Read the model definition and answer for the solid it produces. Units are mm, in the model's axes. Face numbers are marked on the shaded views. A direction names the side the tool comes from. Give positions to 0.01 mm unless a question says otherwise; leave off trailing zeros. Order: outer loops, then holes, each group sorted by start corner. A loop starts at its lowest first (then second) coordinate and runs counter-clockwise, first axis right, second up. Notation, with made-up numbers: (73, 54) - (132, 54) arc R22 ccw to (132, 73) - close; hole circle Ø1 at (20, -11). An arc over 180 degrees is marked (long way). Write each question's results on one line, items separated by ' | '.
Autodesk Inventor part; units mm, degrees
ref_plane "YZ Plane" through (0, 0, 0) normal (1, 0, 0) x (0, 1, 0)
ref_plane "XZ Plane" through (0, 0, 0) normal (0, 1, 0) x (-1, 0, 0)
ref_plane "XY Plane" through (0, 0, 0) normal (0, 0, 1) x (1, 0, 0)
sketch "Sketch1" plane through (0, 0, 0) normal (0, 1, 0) x (-1, 0, 0)
  circle A0 centre (0, 0) radius 5.5
  dimension "d0" = 11
extrude "Extrusion1" add sketch "Sketch1" along normal blind 33
sketch "Sketch6" plane through (0, 0, 0) normal (0, -1, 0) x (1, 0, 0)
  circle A0 centre (0, 0) radius 5.5
  line L0 (3.45, 0) -> (3.45, -4.2834)
  line L1 (0.45, 0) -> (0.45, -5.4816)
  line L2 (3.45, -5.4816) -> (3.45, -4.2834)
  line L3 (3.45, -5.4816) -> (0.45, -5.4816)
  line L4 (0.45, 0) -> (0.45, 5.4816)
  line L5 (3.45, 5.3243) -> (3.45, 0)
  line L6 (3.45, 5.3243) -> (0.45, 5.4816)
  line L7 (0, -5.5) -> (0, 5.5)
  line L8 (-3.45, 0) -> (-3.45, -4.2834)
  line L9 (-0.45, 0) -> (-0.45, -5.4816)
  line L10 (-3.45, -5.4816) -> (-3.45, -4.2834)
  line L11 (-3.45, -5.4816) -> (-0.45, -5.4816)
  line L12 (-0.45, 0) -> (-0.45, 5.4816)
  line L13 (-3.45, 5.3243) -> (-3.45, 0)
  line L14 (-3.45, 5.3243) -> (-0.45, 5.4816)
  point P0 (-3.45, 4.2834)
  point P1 (3.45, 4.2834)
  dimension "d20" = 3
  dimension "d21" = 3
  dimension "d22" = 0.45
  dimension "d23" = 2.05
  dimension "d24" = 2.05
extrude "Extrusion5" add sketch "Sketch6" along normal blind 6 contours A0 L5 L0 L1 L4 | L12 L9 A0 L8 L13
sketch "Sketch8" plane through (0, 0, 0) normal (1, 0, 0) x (0, 1, 0)
  line L0 (0, -5.5) -> (33, -5.5)
  line L1 (0, -5.4816) -> (-6, -5.4816)
  line L2 (0, -5.4816) -> (0, 5.4816)
  line L3 (0, -5.4816) -> (-6, 0.5184)
  line L4 (0, -5.4816) -> (8.4853, -5.4816) construction
  line L5 (-6, -5.4816) -> (-6, 5.4816)
  line L6 (-6, 0.5184) -> (-6, -5.4816)
  point P0 (0, 0)
  dimension "d27" = 135
extrude "Extrusion6" cut sketch "Sketch8" along normal through all both and the other way through all
sketch "Sketch10" plane through (0, 0, 0) normal (1, 0, 0) x (0, 1, 0)
  circle A0 centre (-3.5, 0) radius 1
  line L0 (0, -5.5) -> (33, -5.5)
  line L1 (-6, 0.5184) -> (-6, 5.4816)
  point P0 (0, 0)
  dimension "d30" = 2
  dimension "d31" = 5.5
  dimension "d32" = 2.5
extrude "Extrusion7" cut sketch "Sketch10" along normal through all both and the other way through all
sketch "Sketch11" plane through (0, 33, 0) normal (0, 1, 0) x (1, 0, 0)
  circle A0 centre (0, 3) radius 1
  circle A1 centre (0, -3) radius 1
  point P0 (0, 0)
  dimension "d35" = 2
  dimension "d36" = 2
  dimension "d37" = 3
  dimension "d38" = 3
extrude "Extrusion8" cut sketch "Sketch11" against normal blind 33
properties part number "Part4 finger(indexx)"
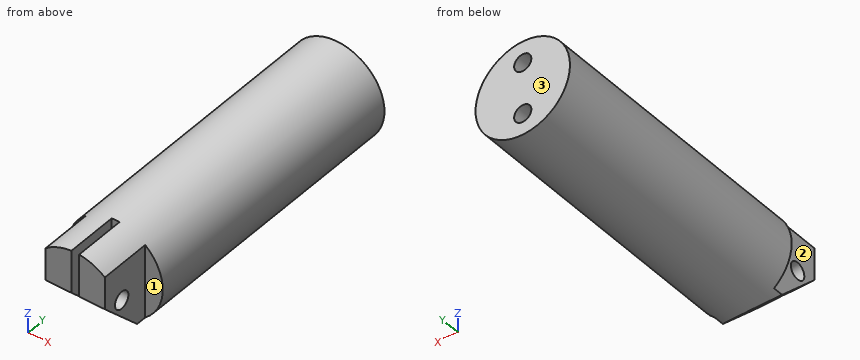
(1) Section D-D (y = 27) is taken. Give the vertices of the cut face in (x, z).
Conclusion:
outline: circle Ø11 at (0, 0); hole circle Ø2 at (0, -3); hole circle Ø2 at (0, 3)
(2) Section B-B (z = -3) is taken. Give the vertices of the cut face in (x, y).
Conclusion:
outline: (-4.61, 0) - (-3.45, 0) - (-3.45, -2.48) - (-0.45, -2.48) - (-0.45, 0) - (-1, 0) - (-1, 33) - (-4.61, 33) - close; (0.45, -2.48) - (3.45, -2.48) - (3.45, 0) - (4.61, 0) - (4.61, 33) - (1, 33) - (1, 0) - (0.45, 0) - close
(3) Consider probe 1 along Z at (x, y) = (0, 22); probe 2 along X at (y, z) = (-1, -1); probe 3 along Y at (x, z) = (3.25, 0). Determine where each line is inside the solid, lowest interval first. Write a range as [from, to].
Conclusion:
probe 1: [-5.5, -4], [-2, 2], [4, 5.5] | probe 2: [-3.45, -0.45], [0.45, 3.45] | probe 3: [-5.48, -4.5], [-2.5, 33]
(4) For the marked faces 1, 2 and 3, determine the directions among +Z, -Z, +X, -X, +Y, -Y from which every point of the face is accessible in a straight line to the end or side of a thin tool.
Conclusion:
face 1: +Z, -Z, +X, -Y | face 2: +Z, -Z, -X, -Y | face 3: +Z, -Z, +X, -X, +Y
(5) Section C-C (y = -3.5) is taken. Give the vertices of the cut face in (x, z), plus the area to 3 significant figures.
Conclusion:
outline: (-3.45, -1.98) - (-0.45, -1.98) - (-0.45, -1) - (-3.45, -1) - close; (-3.45, 1) - (-0.45, 1) - (-0.45, 5.48) arc R5.5 ccw to (-3.45, 4.28) - close; (0.45, -1.98) - (3.45, -1.98) - (3.45, -1) - (0.45, -1) - close; (0.45, 1) - (3.45, 1) - (3.45, 4.28) arc R5.5 ccw to (0.45, 5.48) - close | area: 30.2 mm^2
(6) Section A-A (z = 0) is taken. Give the vertices of the cut face in (x, y), plus the area to 3 significant figures.
Conclusion:
outline: (-5.5, 0) - (-3.45, 0) - (-3.45, -2.5) - (-0.45, -2.5) - (-0.45, 0) - (0.45, 0) - (0.45, -2.5) - (3.45, -2.5) - (3.45, 0) - (5.5, 0) - (5.5, 33) - (-5.5, 33) - close; (-3.45, -5.48) - (-0.45, -5.48) - (-0.45, -4.5) - (-3.45, -4.5) - close; (0.45, -5.48) - (3.45, -5.48) - (3.45, -4.5) - (0.45, -4.5) - close | area: 384 mm^2
(7) Each of these flat-tipped pins is pushed along its axis until it touches: pin 1 (2.5 mm diameter, centred on y = -3.5, z = 0, fed in from +X); pin 2 (3 mm diameter, centred on y = 8.5, z = -3, fed in from +X); pin 3 (1.8 mm diameter, centred on y = -3.5, z = 1, fed in from -X); pin 4 (1.8 mm diameter, centred on y = -3.5, z = 0, fed in from +X). Where does it stop, or does it pass through?
Conclusion:
pin 1: x = 3.45 | pin 2: x = 5.29 | pin 3: x = -3.45 | pin 4: through
